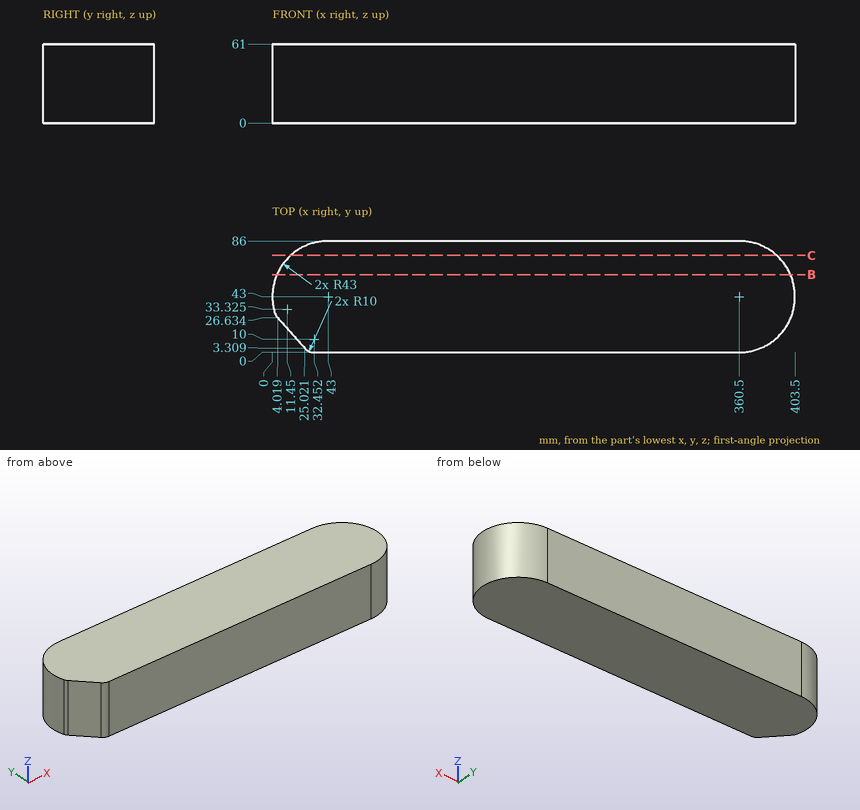
Verification items for this drawing (mm, ordinates from the low corner). Coordinates: 2 decimals unless noted, no trailing zeros. Loops run counter-clockwise (first coordinate to the right, second up) from the corner with the lowest first, then second, coordinate; pieces in that order, holes last. Notation, with made-up numbers: (18, 52.5) -> (34, 52.5) arc R20 ccw to (34, 76.5) -> close; hole circle Ø9 at (-0.5, -6). An arc over 180 degrees is marked (long way). Put each result on its own line as item: value.
1. Section check C-C, the plane y = 75. Record the boundary of the cut face in (x, z).
Result set:
outline: (14.28, 0) -> (389.22, 0) -> (389.22, 61) -> (14.28, 61) -> close
2. Section check B-B, the plane y = 60. Record the boundary of the cut face in (x, z), then the cut area to 3 significant figures.
Result set:
outline: (3.5, 0) -> (400, 0) -> (400, 61) -> (3.5, 61) -> close
area: 24,200 mm^2
3. Thickness scan on line 1 (X direction, y = 7, z = 31) (1 decimal); line 2 (X direction, y = 19, z = 21); line 3 (Y direction, x = 19.5, z = 6). Record the ranges inside material, lowest first.
Result set:
line 1: x = 21.7 to 384
line 2: x = 10.89 to 396.18
line 3: y = 9.44 to 79.01
4. Gauge pin test, flat ends, axial feed: P1, Ø1.5, axis at y = 42.5, z = 36, coming from the +X side; P2, Ø8, axis at y = 57, z = 25, coming from the +X side; P3, Ø4, axis at y = 36.5, z = 49.5, coming from the -X side. Record the tip position at first contact, or that the pin passes through.
Result set:
P1: stops at x = 403.5
P2: stops at x = 402.32
P3: stops at x = 0.24
